CAD build for the part. Positions are in the model's coordinates, mm. A direction names the side the tool comes from. Round coordinates to 2 decimals unless told otherwise and drop trailing zeros. Loops run counter-clockwise (first coordinate to the right, second up) from the corner with the lowest first, then second, coordinate; pieces in that order, holes last.
from build123d import *

# Parameters (mm, degrees)
F0_W          = 90
F0_H          = 52
F1_DEPTH      = 16
F3_DEPTH      = 1323
F0_W_2        = 2.3
F0_H_2        = 10
F4_DEPTH      = 12.2
F5_R          = 2.65
F6_DEPTH      = 100
F6_DEPTH_BACK = 25
F7_DEPTH      = 2
F8_R          = 7
F9_R          = 0.9


with BuildPart() as f1:
    # F0 (on Top) → F1 (new body)
    with BuildSketch(Plane.XY):
        Rectangle(F0_W, F0_H)
        Polygon((-42.75, 23.75), (42.75, 23.75), (42.75, -23.75), (38.55, -23.75), (36.25, -23.75), (-36.25, -23.75), (-38.55, -23.75), (-42.75, -23.75), align=None, mode=Mode.SUBTRACT)
    extrude(amount=F1_DEPTH)

    # F2 (on face) → F3 (cut)
    with BuildSketch(Plane(origin=(-45, 0, 0), x_dir=(0, -1, 0), z_dir=(-1, 0, 0))):
        Polygon((-26, 16), (-26, 3), (-23.75, 3), (23.75, 13.75), (23.75, 16), align=None)
    extrude(amount=-F3_DEPTH, mode=Mode.SUBTRACT)

    # F0 (on Top) → F4 (join)
    with BuildSketch(Plane.XY):
        with Locations((-37.4, -18.75)):
            Rectangle(F0_W_2, F0_H_2)
        with Locations((37.4, -18.75)):
            Rectangle(F0_W_2, F0_H_2)
    extrude(amount=F4_DEPTH)

    # F5 (on face) → F6 (cut, two sides)
    with BuildSketch(Plane(origin=(-38.55, 0, 0), x_dir=(0, -1, 0), z_dir=(-1, 0, 0))) as f6_sk:
        with Locations((19.05, 7)):
            Circle(F5_R)
    extrude(amount=-F6_DEPTH, mode=Mode.SUBTRACT)
    extrude(f6_sk.sketch, amount=F6_DEPTH_BACK, mode=Mode.SUBTRACT)

    # F0 (on Top) → F7 (join)
    with BuildSketch(Plane.XY):
        Rectangle(F0_W, F0_H)
        Polygon((-42.75, 23.75), (42.75, 23.75), (42.75, -23.75), (38.55, -23.75), (36.25, -23.75), (-36.25, -23.75), (-38.55, -23.75), (-42.75, -23.75), align=None, mode=Mode.SUBTRACT)
        Polygon((42.75, -23.75), (42.75, 23.75), (-42.75, 23.75), (-42.75, -23.75), (-38.55, -23.75), (-38.55, -13.75), (-36.25, -13.75), (-36.25, -23.75), (36.25, -23.75), (36.25, -13.75), (38.55, -13.75), (38.55, -23.75), align=None)
    extrude(amount=F7_DEPTH)

    # F8
    f8_edges = [f1.edges().sort_by_distance(p)[0] for p in [
        (-37.4, -13.75, 12.2),
        (37.4, -13.75, 12.2),
    ]]
    fillet(f8_edges, radius=F8_R)

    # F9
    f9_edges = [f1.edges().sort_by_distance(p)[0] for p in [
        (0, -26, 16),
        (0, -23.75, 16),
        (0, 23.75, 3),
        (0, 26, 3),
    ]]
    fillet(f9_edges, radius=F9_R)


solid = f1.part
Item 1: Cut at D-D (y = -4). List the corners of the cut face in (x, z), plus the area to 3 significant figures.
Verdict:
outline: (-45, 0) - (45, 0) - (45, 9.28) - (42.75, 9.28) - (42.75, 2) - (-42.75, 2) - (-42.75, 9.28) - (-45, 9.28) - close
area: 213 mm2
Item 2: Flat gauge pins, fed straight in: P1, Ø3, axis at y = -19.05, z = 7, coming from the -X side; P2, Ø8, axis at x = -13.5, z = 9.5, coming from the +Y side; P3, Ø1.5, axis at x = 2.5, y = -20, coming from the +Z side; P4, Ø0.7, axis at x = 37.5, z = 4, coming from the +Y side. Where does each tip first touch, or does it go through?
Verdict:
P1: passes through
P2: stops at y = -23.75
P3: stops at z = 2
P4: stops at y = -13.75
Item 3: 3-axis set-ups, long thin cutter, end or side, ignore diameter. For faces 1 (the flat face through (38.55, -21, 4.8)), 2 (the cylindrical face through (37.42, -15.85, 10.2)), 3 (the cylindrical face through (43.859, -16.947, 5.388)): which of +Z, -Z, +X, -X, +Y, -Y reach the whole face in a straight line?
Verdict:
face 1: +Z
face 2: +Z, +Y
face 3: +X, -X
Item 4: Cut at A-A (x = -16). List the corners of the cut face in (y, z).
Verdict:
outline: (-26, 0) - (26, 0) - (26, 2.1) arc R0.9 ccw to (25.1, 3) - (24.65, 3) arc R0.9 ccw to (23.75, 2.1) - (23.75, 2) - (-23.75, 2) - (-23.75, 15.1) arc R0.9 ccw to (-24.65, 16) - (-25.1, 16) arc R0.9 ccw to (-26, 15.1) - close
Item 5: Mould opens along Y. For faces 4 (the flat face through (-1, 0, 0)), 5 (the flat face through (37, -13.75, 4)), 6 (the cylindrical face through (-37.38, -15.85, 10.2)) say: released by +Y, released by -Y, zero draft, split by the parting line, or undercut.
Verdict:
face 4: zero draft
face 5: undercut
face 6: released by +Y
Item 6: Wall check: L1, parallel to X at y = -21.5, z = 12.5; L2, parallel to Z at x = 29, y = -4.5; L3, parallel to Y at x = -6, z = 11.5. Give the ranges that are in metal, low to high.
Verdict:
L1: x = -45 to -42.75, 42.75 to 45
L2: z = 0 to 2
L3: y = -26 to -23.75
Item 7: Cut at B-B (y = -19.05). State how many separate pieces and enclosed holes the cut face has, plus the area to 3 significant figures.
Verdict:
separate pieces: 5
enclosed holes: 0
area: 226 mm2
